```python
from build123d import *

# Parameters (mm, degrees)
F0_W     = 750
F0_H     = 700
F0_R     = 30
F0_R_2   = 4.25
F0_R_3   = 6
F1_DEPTH = 150
F2_DEPTH = 130
F3_DEPTH = 40
F6_R     = 50.5
F6_R_2   = 30
F7_DEPTH = 75


with BuildPart() as f1:
    # F0 (on Top) → F1 (new body)
    with BuildSketch(Plane.XY):
        Rectangle(F0_W, F0_H)
        with Locations((-300, -275)):
            Circle(F0_R, mode=Mode.SUBTRACT)
        with Locations((-97.427858, -56.25)):
            Circle(F0_R_2, mode=Mode.SUBTRACT)
        with Locations((300, -275)):
            Circle(F0_R, mode=Mode.SUBTRACT)
        with Locations((0, -112.5)):
            Circle(F0_R_2, mode=Mode.SUBTRACT)
        with Locations((97.427858, -56.25)):
            Circle(F0_R_2, mode=Mode.SUBTRACT)
        with Locations((-112.5, 0)):
            Circle(F0_R_3, mode=Mode.SUBTRACT)
        with Locations((-97.427858, 56.25)):
            Circle(F0_R_2, mode=Mode.SUBTRACT)
        with Locations((-300, 275)):
            Circle(F0_R, mode=Mode.SUBTRACT)
        with Locations((112.5, 0)):
            Circle(F0_R_3, mode=Mode.SUBTRACT)
        with Locations((97.427858, 56.25)):
            Circle(F0_R_2, mode=Mode.SUBTRACT)
        with Locations((0, 112.5)):
            Circle(F0_R_2, mode=Mode.SUBTRACT)
        with Locations((300, 275)):
            Circle(F0_R, mode=Mode.SUBTRACT)
        with Locations((-112.5, 0)):
            Circle(F0_R_3)
        with Locations((-97.427858, -56.25)):
            Circle(F0_R_2)
        with Locations((-97.427858, 56.25)):
            Circle(F0_R_2)
        with Locations((0, 112.5)):
            Circle(F0_R_2)
        with Locations((112.5, 0)):
            Circle(F0_R_3)
        with Locations((97.427858, -56.25)):
            Circle(F0_R_2)
        with Locations((0, -112.5)):
            Circle(F0_R_2)
    extrude(amount=-F1_DEPTH)

    # F0 (on Top) → F3 (cut)
    with BuildSketch(Plane.XY):
        with Locations((-112.5, 0)):
            Circle(F0_R_3)
        with Locations((-97.427858, 56.25)):
            Circle(F0_R_2)
        with Locations((0, 112.5)):
            Circle(F0_R_2)
        with Locations((97.427858, 56.25)):
            Circle(F0_R_2)
        with Locations((112.5, 0)):
            Circle(F0_R_3)
        with Locations((97.427858, -56.25)):
            Circle(F0_R_2)
        with Locations((0, -112.5)):
            Circle(F0_R_2)
        with Locations((-97.427858, -56.25)):
            Circle(F0_R_2)
    extrude(amount=-F3_DEPTH, mode=Mode.SUBTRACT)


with BuildPart() as f2:
    # F0 (on Top) → F2 (new body)
    with BuildSketch(Plane.XY):
        Rectangle(F0_W, F0_H)
        with Locations((-300, -275)):
            Circle(F0_R, mode=Mode.SUBTRACT)
        with Locations((-97.427858, -56.25)):
            Circle(F0_R_2, mode=Mode.SUBTRACT)
        with Locations((300, -275)):
            Circle(F0_R, mode=Mode.SUBTRACT)
        with Locations((0, -112.5)):
            Circle(F0_R_2, mode=Mode.SUBTRACT)
        with Locations((97.427858, -56.25)):
            Circle(F0_R_2, mode=Mode.SUBTRACT)
        with Locations((-112.5, 0)):
            Circle(F0_R_3, mode=Mode.SUBTRACT)
        with Locations((-97.427858, 56.25)):
            Circle(F0_R_2, mode=Mode.SUBTRACT)
        with Locations((-300, 275)):
            Circle(F0_R, mode=Mode.SUBTRACT)
        with Locations((112.5, 0)):
            Circle(F0_R_3, mode=Mode.SUBTRACT)
        with Locations((97.427858, 56.25)):
            Circle(F0_R_2, mode=Mode.SUBTRACT)
        with Locations((0, 112.5)):
            Circle(F0_R_2, mode=Mode.SUBTRACT)
        with Locations((300, 275)):
            Circle(F0_R, mode=Mode.SUBTRACT)
    extrude(amount=-F2_DEPTH)


with BuildPart() as f2_1:
    # F4: moved
    add(f2.part.moved(Location((0, 0, -20))))

    # F5: union F1
    add(f1.part)

    # F6 (on face) → F7 (cut)
    with BuildSketch(Plane(origin=(0, 0, -150), x_dir=(1, 0, 0), z_dir=(0, 0, -1))):
        with Locations((-300, 275)):
            Circle(F6_R)
        with Locations((-300, 275)):
            Circle(F6_R_2, mode=Mode.SUBTRACT)
        with Locations((-300, -275)):
            Circle(F6_R)
        with Locations((-300, -275)):
            Circle(F6_R_2, mode=Mode.SUBTRACT)
        with Locations((300, -275)):
            Circle(F6_R)
        with Locations((300, -275)):
            Circle(F6_R_2, mode=Mode.SUBTRACT)
        with Locations((300, 275)):
            Circle(F6_R)
        with Locations((300, 275)):
            Circle(F6_R_2, mode=Mode.SUBTRACT)
    extrude(amount=-F7_DEPTH, mode=Mode.SUBTRACT)


solid = f2_1.part
```
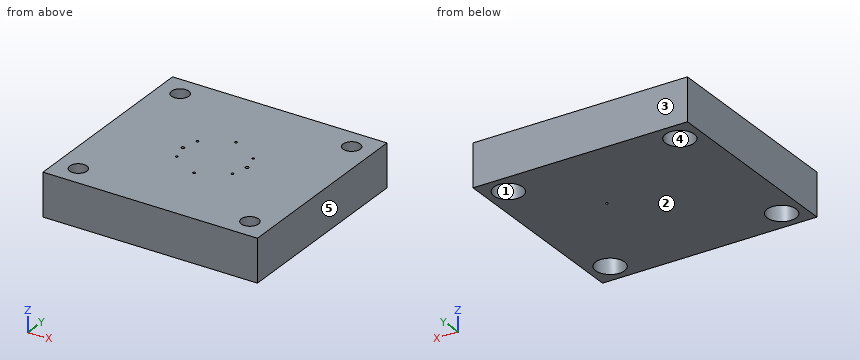
Verification items for the finished model (mm, model axes). Face numbers are marked on the shaded views. A direction names the side the tool comes from. Round coordinates to 2 decimals unless told otherwise and drop trailing zeros. Write each loop counter-clockwise with the first axis right and the second up, starting at its lowest first coordinate (ties: lowest second). Pieces come first, ordered by that corner, then holes.
1. Section check B-B on x = 300. Enter the section's corners in (y, z).
2. Section check C-C on z = -12.5. State how many separate pieces and enclosed holes the cut face has, plus the area to 3 significant figures.
3. Gauge pin test, flat end, axial feed: P1, Ø7, axis at x = 0, y = 112.5, coming from the +Z side. Record the tip position at first contact, or that the pin passes through.
4. Scan lines: L1, parallel to Y at x = -300, z = -46; L2, parallel to X at y = 56, z = -23; L3, parallel to Y at x = 259.5, z = -121. Record each from-to range of solid material in increasing order.
5. Section check D-D on x = -258. Enter the section's corners in (y, z), plus the area to 3 significant figures.
6. Draft check along X on the marked faces 3, 4 and 5. Enter one of: +X half, -X half, draft (parallel to the pull), parting line (faces both ways), or undercut.
7. Access from +Z, -Z, +X, -X, +Y, -Y to the whole of each face (thin tool, end or side, straight path). Record for the marked faces 1 and 2.
8. Section check A-A on y = -275. Enter the section's corners in (x, z).
Answer:
1. outline: (-350, -150) - (-325.5, -150) - (-325.5, -75) - (-305, -75) - (-305, 0) - (-350, 0) - close; (-245, -75) - (-224.5, -75) - (-224.5, -150) - (224.5, -150) - (224.5, -75) - (245, -75) - (245, 0) - (-245, 0) - close; (305, -75) - (325.5, -75) - (325.5, -150) - (350, -150) - (350, 0) - (305, 0) - close
2. separate pieces: 1
2. enclosed holes: 12
2. area: 513,000 mm2
3. P1: stops at z = -40
4. L1: y = -350 to -305, -245 to 245, 305 to 350
4. L2: x = -375 to -101.67, -93.19 to 93.19, 101.67 to 375
4. L3: y = -350 to -305.17, -244.83 to 244.83, 305.17 to 350
5. outline: (-350, -150) - (-303.04, -150) - (-303.04, -75) - (-246.96, -75) - (-246.96, -150) - (246.96, -150) - (246.96, -75) - (303.04, -75) - (303.04, -150) - (350, -150) - (350, 0) - (-350, 0) - close
5. area: 96,600 mm2
6. face 3: draft
6. face 4: undercut
6. face 5: +X half
7. face 1: -Z
7. face 2: -Z, +X, -X, +Y, -Y
8. outline: (-375, -150) - (-350.5, -150) - (-350.5, -75) - (-330, -75) - (-330, 0) - (-375, 0) - close; (-270, -75) - (-249.5, -75) - (-249.5, -150) - (249.5, -150) - (249.5, -75) - (270, -75) - (270, 0) - (-270, 0) - close; (330, -75) - (350.5, -75) - (350.5, -150) - (375, -150) - (375, 0) - (330, 0) - close
